Can you work these out from the model? Positions are in its coordinate system, mm. A direction names the side the tool comes from. Round coordinates to 2 decimals unless told otherwise and drop trailing zeros. Write each loop counter-clockwise with the first axis right and the second up, starting at its lowest first coordinate (ties: lowest second). Pieces come first, ordered by that corner, then holes.
Q1. If we section it at B-B (y = -55): Please give me the cut outline in (x, z).
Q2. We'd pull the mould along Y, two halves only. Please class faces 1 (the flat face through (25.333, -16.374, 163.015)), 2 (the cylindrical face through (16.32, 22.75, 162.94)), 3 (the cylindrical face through (-26.577, -8.813, 162.945)): +Y half, -Y half, draft (parallel to the pull), parting line (faces both ways), or undercut.
Q3. If we section it at D-D (z = 29.5): Please give me the cut outline in (x, y).
Q4. I'm going to push flat-ended pins straight in: pin 1 Ø1.5 at (x, z) = (9.5, 47.5) entering from -Y; pin 2 Ø2 at (x, z) = (12.5, 162) entering from +Y; pin 3 Ø12 at (y, z) = (25.5, 83.5) entering from +X. Where does each tip first touch, or does it pass through?
Q5. For faces 4 (the flat face through (7.406, -29.269, 163.015)), 5 (the flat face through (-25.55, -16.09, 163.01)), 6 (the flat face through (-28.18, 10.75, 163.01)), 7 (the flat face through (-29.05, 8.22, 163.01)), 8 (the cylindrical face through (27.83, 3.09, 162.94)), which set-ups out of +Z, -Z, +X, -X, +Y, -Y let a thin tool reach every point of the face, with its end or its side?
Q6. If we section it at A-A (z = 150.5): Please give me the cut outline in (x, y), plus the area to 3 significant figures.
Q7. Please list where these lines run through material, in increasing order: line 1 along Z through (x, y) = (-2, 35.5); line 2 along X through (y, z) = (1, 193.5); line 3 along X through (y, z) = (10, 89).
Q8. If we section it at C-C (x = -43): Please give me the cut outline in (y, z).
from build123d import *

# Parameters (mm, degrees)
SKETCH1_R           = 75
BOSS_EXTRUDE1_DEPTH = 137
SKETCH2_R           = 10
BOSS_EXTRUDE2_DEPTH = 70
SKETCH4_R           = 28
BOSS_EXTRUDE3_DEPTH = 5
BOSS_EXTRUDE4_DEPTH = 5
CIRPATTERN1_COUNT   = 15


with BuildPart() as part:
    # Sketch1 → Boss-Extrude1 (new body)
    with BuildSketch(Plane.XY):
        Circle(SKETCH1_R)
    extrude(amount=BOSS_EXTRUDE1_DEPTH)

    # Sketch2 → Boss-Extrude2 (add)
    with BuildSketch(Plane.XY.offset(137)):
        Circle(SKETCH2_R)
    extrude(amount=BOSS_EXTRUDE2_DEPTH)

    # Sketch4 → Boss-Extrude3 (add)
    with BuildSketch(Plane.XY.offset(160.48)):
        Circle(SKETCH4_R)
    extrude(amount=BOSS_EXTRUDE3_DEPTH)

    # Sketch5 → Boss-Extrude4 (add)
    with BuildSketch(Plane.XY.offset(165.48)):
        Polygon((3.567039891, 25.329459933), (0.529235594, 32.424417196), (-4.096275486, 26.246122872), align=None)
    boss_extrude4 = extrude(amount=-BOSS_EXTRUDE4_DEPTH)

    # CirPattern1: Boss-Extrude4 ×15 about axis
    cirpattern1_axis = Axis((0, 0, 0), (0, 0, 1))
    for i in range(1, CIRPATTERN1_COUNT):
        add(boss_extrude4.rotate(cirpattern1_axis, i * 360 / CIRPATTERN1_COUNT))


solid = part.part
A:
1. outline: (-50.99, 0) - (50.99, 0) - (50.99, 137) - (-50.99, 137) - close
2. face 1: -Y half
2. face 2: +Y half
2. face 3: undercut
3. outline: circle Ø150 at (0, 0)
4. pin 1: stops at y = -74.49
4. pin 2: stops at y = 29.31
4. pin 3: stops at x = 72.42
5. face 4: +Z, +X, -Y
5. face 5: +Z, -X, -Y
5. face 6: +Z, -X, +Y
5. face 7: +Z, -X
5. face 8: +Z, +X
6. outline: circle Ø20 at (0, 0)
6. area: 314 mm2
7. line 1: z = 0 to 137
7. line 2: x = -9.95 to 9.95
7. line 3: x = -74.33 to 74.33
8. outline: (-61.45, 0) - (61.45, 0) - (61.45, 137) - (-61.45, 137) - close
